```python
from build123d import *

# Parameters (mm, degrees)
F1_DEPTH = 63.5
F0_W     = 25.4
F0_H     = 19.05
F0_H_2   = 4.7498
F0_H_3   = 4.7752
F2_DEPTH = 25.4
F3_DEPTH = 3.175
F5_R     = 19.0095175901
F7_D     = 25.4
F7_DEPTH = 12.7
F7_TIP   = 7.6309298617


with BuildPart() as f1:
    # F0 (on Top) → F1 (new body, symmetric)
    with BuildSketch(Plane.XY):
        Polygon((41.275, -9.525), (41.275, 9.525), (22.225, 9.525), (-41.275, 9.525), (-41.275, -9.525), align=None)
    extrude(amount=F1_DEPTH, both=True)

    # F0 (on Top) → F2 (join, symmetric)
    with BuildSketch(Plane.XY):
        with BuildLine():
            Line((22.225, 9.525), (41.275, 9.525))
            Line((41.275, 9.525), (41.275, 30.3160412997))
            ThreePointArc((41.275, 30.3160412997), (44.9534924173, 39.1967075827), (53.8341587003, 42.8752))
            Line((53.8341587003, 42.8752), (60.325, 42.8752))
            Line((60.325, 42.8752), (60.325, 61.9252))
            Line((60.325, 61.9252), (53.8341587003, 61.9252))
            add(Edge.make_bspline(
                [(52.4478102945, 61.8947833874), (52.9089875046, 61.9054541447), (53.3711097525, 61.9155870845), (53.8341587003, 61.9252)],
                knots=[107.6548099731, 107.6548099731, 107.6548099731, 107.6548099731, 108.5888255242, 108.5888255242, 108.5888255242, 108.5888255242], degree=3))
            ThreePointArc((52.4478102945, 61.8947833874), (30.9982196949, 52.1714480331), (22.225, 30.3160412997))
            Line((22.225, 30.3160412997), (22.225, 9.525))
        make_face()
        with Locations((73.025, 52.4002)):
            Rectangle(F0_W, F0_H)
        with Locations((73.025, 64.3001)):
            Rectangle(F0_W, F0_H_2)
        with Locations((73.025, 40.4876)):
            Rectangle(F0_W, F0_H_3)
    extrude(amount=F2_DEPTH, both=True)

    # F0 (on Top) → F3 (join, symmetric)
    with BuildSketch(Plane.XY):
        with BuildLine():
            Line((-41.275, 9.525), (22.225, 9.525))
            Line((22.225, 9.525), (22.225, 30.3160412997))
            ThreePointArc((22.225, 30.3160412997), (30.9982196949, 52.1714480331), (52.4478102945, 61.8947833874))
            add(Edge.make_bspline(
                [(-41.275, 9.525), (-41.3081932608, 52.2900973959), (-0.7075626129, 60.6648698646), (52.4478102945, 61.8947833874)],
                knots=[0, 0, 0, 0, 107.6548099731, 107.6548099731, 107.6548099731, 107.6548099731], degree=3))
        make_face()
    extrude(amount=F3_DEPTH, both=True)

    # F0 (on Top) → F4 (revolve)
    with BuildSketch(Plane.XY):
        Polygon((85.725, 61.9252), (85.725, 42.8752), (85.725, 38.1), (111.125, 38.1), (111.125, 66.675), (85.725, 66.675), align=None)
    revolve(axis=Axis((85.725, 52.3875, 0), (0, 1, 0)))

    # F5
    f5_edges = [f1.edges().sort_by_distance(p)[0] for p in [
        (111.125, 66.675, 0),
    ]]
    fillet(f5_edges, radius=F5_R)

    # F7
    with Locations(Plane.XZ.offset(-38.1)):
        with Locations((85.725, 0)):
            Hole(F7_D / 2, depth=F7_DEPTH)
            with Locations((0, 0, -(F7_DEPTH + F7_TIP / 2))):  # 118° drill point
                Cone(0, F7_D / 2, F7_TIP, mode=Mode.SUBTRACT)


solid = f1.part
```
The model under review builds one solid part; all positions refer to its coordinate system, in mm. A direction names the side the tool comes from. Give positions to 0.01 mm unless a question says otherwise; leave off trailing zeros. Write each loop counter-clockwise with the first axis right and the second up, starting at its lowest first coordinate (ties: lowest second). Pieces come first, ordered by that corner, then holes.
(1) To check wall thickness, follow L1, parallel to Y at x = -23, z = 11.5 (3 decimals); L2, parallel to X at y = 14, z = -9.5 (3 decimals); L3, parallel to Z at x = -18, y = 47 (3 decimals). State the ranges of each line that lie inside material, in increasing order.
(2) The part is to be moulded in two halves that separate along Z. For faces 5 (the flat face through (1, 9.525, 34)), 6 (the flat face through (-6, 30, 3.175)), 7 (the cylindrical face through (73.61, 44.54, 3.81)), say which applies: released by +Z, released by -Z, zero draft, split by the parting line, or undercut.
(3) Tool access review of faces 1 (the flat face through (80, 38.1, -12)), 2 (the flat face through (39, 33, -25.4)), 3 (the flat face through (57, 42.875, 0)), 4 (the flat face through (-6, 30, -3.175)): name each direction out of +Z, -Z, +X, -X, +Y, -Y from which nothing blocks a thin tool from reaching the whole face with its end or side.
(4) For P1, Ø23, axis at y = 15.5, z = -18.5, coming from the -X side (3 decimals); P2, Ø2, axis at x = 23.5, y = 16.5, coming from the +Z side; P3, Ø18, axis at x = 8.5, z = 44, coming from the +Y side (3 decimals); P4, Ø4, axis at x = 2.5, y = 56, coming from the +Z side (3 decimals), all flat-tipped, find the tip position at first contact; note any pin that passes through.
(5) Consider section A-A, the plane z = 32.5. Give the boundary of the cut face in (x, y) (3 decimals).
Returned:
1. L1: y = -9.525 to 9.525
1. L2: x = 22.225 to 41.275
1. L3: z = -3.175 to 3.175
2. face 5: zero draft
2. face 6: released by +Z
2. face 7: undercut
3. face 1: +Z, -Z, +X, -Y
3. face 2: -Z, +X, -X, +Y
3. face 3: +Z, -Z, -Y
3. face 4: -Z, -X, +Y
4. P1: stops at x = -41.275
4. P2: stops at z = 25.4
4. P3: stops at y = 9.525
4. P4: stops at z = 3.175
5. outline: (-41.275, -9.525) - (41.275, -9.525) - (41.275, 9.525) - (-41.275, 9.525) - close
